Autodesk Inventor part; units mm, degrees
ref_plane "YZ Plane" through (0, 0, 0) normal (1, 0, 0) x (0, 1, 0)
ref_plane "XZ Plane" through (0, 0, 0) normal (0, 1, 0) x (-1, 0, 0)
ref_plane "XY Plane" through (0, 0, 0) normal (0, 0, 1) x (1, 0, 0)
sketch "Sketch1" plane through (0, 0, 0) normal (0, 1, 0) x (-1, 0, 0)
  line L0 (0, 0) -> (42, 0)
  line L1 (42, 0) -> (42, -13)
  line L2 (42, -13) -> (38, -13)
  line L3 (38, -13) -> (38, -11)
  line L4 (38, -11) -> (0, -11)
  line L5 (0, -11) -> (0, 0)
  dimension "d0" = 22
  dimension "d1" = 38
  dimension "d2" = 26
  dimension "d3" = 4
revolve "Revolution1" add sketch "Sketch1" angle 360 about axis through (0, 0, 0) along (-1, 0, 0)
sketch "Sketch3" plane through (0, 0, 0) normal (0, 1, 0) x (-1, 0, 0)
  line L0 (0, 0) -> (42, 0)
  line L1 (42, 13) -> (42, -13)
  line L2 (0, 0) -> (0, 4)
  line L3 (0, 11) -> (0, -11)
  line L4 (0, 4) -> (5, 4)
  line L5 (5, 4) -> (5, 2)
  line L6 (5, 2) -> (10, 2)
  line L7 (10, 2) -> (10, 2.75)
  line L8 (10, 2.75) -> (42, 2.75)
  dimension "d16" = 5.5
  dimension "d17" = 8
  dimension "d18" = 4
  dimension "d19" = 5
  dimension "d20" = 5
revolve "Revolution2" cut sketch "Sketch3" angle 360 about axis through (0, 0, 0) along (-1, 0, 0)
pattern_linear "Rectangular Pattern1" count 2 spacing 6 along (0, 0, 1) of "Revolution2"
pattern_linear "Rectangular Pattern2" count 2 spacing 6 along (0, 0, -1) of "Revolution2"
sketch "Sketch4" plane through (0, 0, 0) normal (1, 0, 0) x (0, 0, -1)
  arc A0 (-3, 2.6458) -> (-3, -2.6458) centre (-6, 0) ccw construction
  arc A1 (3, -2.6458) -> (3, 2.6458) centre (6, 0) ccw construction
  circle A2 centre (-6, 0) radius 2
  circle A3 centre (6, 0) radius 2
  line L0 (-6, 0) -> (6, 0) construction
  line L1 (-6, -4) -> (6, -4)
  line L2 (6, 4) -> (-6, 4)
  arc A4 (-6, 4) -> (-6, -4) centre (-6, 0) ccw
  arc A5 (6, -4) -> (6, 4) centre (6, 0) ccw
  point P0 (0, 0)
  point P1 (0, 0)
extrude "Extrusion1" cut sketch "Sketch4" against normal up to surface (5 mm away) contours A2 | A3 | A4 L2 A5 L1
properties part number "029" material "Acetal Resin, White"
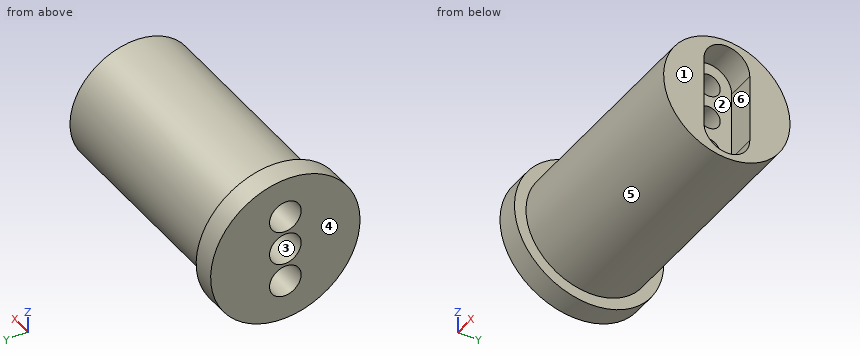
Can you work these out from the model? Positions are in its coordinate system, mm. Face numbers are marked on the shaded views. A direction names the side the tool comes from. Coordinates: 2 decimals unless noted, no trailing zeros. Order: outer loops, then holes, each group sorted by start corner. A loop starts at its lowest first (then second) coordinate and runs counter-clockwise, first axis right, second up. Notation, with made-up numbers: (-29.5, 15) - (-18.5, 15) arc R22 ccw to (-18.5, 49) - close; hole circle Ø8 at (35.5, 72.5). An arc over 180 degrees is marked (long way). Answer as a JSON object with one key per item and string values. Group by question number.
Q1. Imagine slicing it at D-D (x = -19). Please give me the cut outline in (y, z).
Q2. Will these pins go through, and if not, where does the flat tip stop? P1, Ø1.6, axis at y = -1, z = 1, coming from the -X side; P2, Ø2.5, axis at x = -2.5, z = 2, coming from the -Y side; P3, Ø3, axis at x = -8.5, y = 2.5, coming from the -Z side.
Q3. Imagine slicing it at B-B (y = 0). Give the number of separate pieces and of enclosed holes in the cut face, and give its area (3 significant figures).
Q4. Imagine slicing it at C-C (x = -3.5). Please give me the cut outline in (y, z).
Q5. I need wall thicknesses on line 1 (Z direction, x = -15.5, y = -1); line 2 (Y direction, x = -24, z = 0); line 3 (Y direction, x = -6.6, z = 0). Which ranges of each line are inside material? Lowest first, please. Write a range as from..to.
Q6. We'd pull the mould along Y, two halves only. Please class the marked faces 4, 5 and 6: +Y half, -Y half, draft (parallel to the pull), parting line (faces both ways), or undercut.
Q7. Imagine slicing it at A-A (z = 0). Please give me the cut outline in (x, y).
Q8. On a 3-axis mill with a long thin cutter (end or side, diameter ignored), from which of +Z, -Z, +X, -X, +Y, -Y can I reach the whole of each face in a straight line? I mean the marked faces 1, 2 and 3. Say none if no direction works.
Determined:
{
 "1": {"outline": "circle Ø22 at (0, 0); hole circle Ø5.5 at (0, -6); hole circle Ø5.5 at (0, 0); hole circle Ø5.5 at (0, 6)"},
 "2": {"P1": "stops at x = -10", "P2": "stops at y = -10.97", "P3": "stops at z = -10.95"},
 "3": {"separate pieces": "4", "enclosed holes": "0", "area": "252 mm2"},
 "4": {"outline": "circle Ø22 at (0, 0); hole (-4, -6) arc R4 ccw to (4, -6) - (4, 6) arc R4 ccw to (-4, 6) - close"},
 "5": {"line 1": "z = -10.95..-8.56, -3.44..-2.56, 2.56..3.44, 8.56..10.95", "line 2": "y = -11..-2.75, 2.75..11", "line 3": "y = -11..-2, 2..11"},
 "6": {"face 4": "draft", "face 5": "parting line", "face 6": "undercut"},
 "7": {"outline": "(-42, -13) - (-38, -13) - (-38, -11) - (0, -11) - (0, -4) - (-5, -4) - (-5, -2) - (-10, -2) - (-10, -2.75) - (-42, -2.75) - close; (-42, 2.75) - (-10, 2.75) - (-10, 2) - (-5, 2) - (-5, 4) - (0, 4) - (0, 11) - (-38, 11) - (-38, 13) - (-42, 13) - close"},
 "8": {"face 1": "+Z, -Z, +X, +Y, -Y", "face 2": "+X", "face 3": "-X"}
}
